CAD build for the part. Positions are in the model's coordinates, mm. A direction names the side the tool comes from. Round coordinates to 2 decimals unless told otherwise and drop trailing zeros. Loops run counter-clockwise (first coordinate to the right, second up) from the corner with the lowest first, then second, coordinate; pieces in that order, holes last. Notation, with made-up numbers: M 14.25,-4.5 L 25.25,-4.5 A23 ccw 25.25,13.5 Z; hole C 16.5,-30 d7. An arc over 180 degrees is marked long. Use a Markdown table: item, result. Add a question column.
(1) Band-saw the part on D-D, the plane z = 10.75. Give the number of separate pieces and of enclosed holes in the cut face, and give its area (3 significant figures).
(2) Flat gauge pins, fed straight in: P1, Ø3, axis at x = -8.5, y = -8.5, coming from the +Z side; P2, Ø2, axis at x = -14, z = 9.5, coming from the -Y side; P3, Ø5, axis at y = -9, z = 7, coming from the +X side. Where does each tip first touch, or does it go through?
(3) Band-saw the part on C-C, the plane y = 15. Write the cut outline in (x, z).
(4) Which spindle directions (+Z, -Z, +X, -X, +Y, -Y) get a long thin tool onto all of the face, cutting with end or side? Do faces 1 (the face through (9, -8.16, 1.87)), 2 (the face through (-23.65, -12.07, 4.76)), 3 (the face through (0.6, 9.7, 3.8)). Say none if no direction does.
(5) Wall check: L1, parallel to X at y = -0.5, z = 2; L2, parallel to X at y = 2, z = 5.5; L3, parallel to Y at x = 0.5, z = 1.25. Give the ranges that are in metal, low to high.
(6) Two-plate mould, pull along X, no slides. Class faces 4 (the face through (-28, 21, 7)), 5 (the face through (0, -7, 11.8)), 6 (the face through (-12.28, -0.06, 1.87)): released by +X, released by -X, zero draft, split by the parting line, or undercut.
(7) Band-saw the part on A-A, the plane y = 0. Write the cut outline in (x, z).
Autodesk Inventor part; units mm, degrees
ref_plane "YZ Plane" through (0, 0, 0) normal (1, 0, 0) x (0, 1, 0)
ref_plane "XZ Plane" through (0, 0, 0) normal (0, 1, 0) x (-1, 0, 0)
ref_plane "XY Plane" through (0, 0, 0) normal (0, 0, 1) x (1, 0, 0)
sketch "Эскиз1" plane through (0, 0, 0) normal (0, 0, 1) x (1, 0, 0)
  circle A0 centre (0, 0) radius 14
  circle A1 centre (-11, 0) radius 1.2813
  circle A2 centre (-7.7782, -7.7782) radius 1.2813
  circle A3 centre (0, -11) radius 1.2813
  circle A4 centre (7.7782, -7.7782) radius 1.2813
  circle A5 centre (11, 0) radius 1.2813
  circle A6 centre (7.7782, 7.7782) radius 1.2813
  circle A7 centre (0, 11) radius 1.2813
  circle A8 centre (-7.7782, 7.7782) radius 1.2813
  circle A9 centre (0, 0) radius 6
  dimension "d3" = 12
extrude "Выдавливание1" add sketch "Эскиз1" along normal blind 1.8
sketch "Эскиз2" plane through (0, 0, 1.8) normal (0, 0, 1) x (1, 0, 0)
  circle A0 centre (0, 0) radius 14
  circle A1 centre (0, 0) radius 6
  circle A2 centre (-7.7782, 7.7782) radius 1.2813
  circle A3 centre (0, 11) radius 1.2813
  circle A4 centre (7.7782, 7.7782) radius 1.2813
  circle A5 centre (11, 0) radius 1.2813
  circle A6 centre (7.7782, -7.7782) radius 1.2813
  circle A7 centre (0, -11) radius 1.2813
  circle A8 centre (-7.7782, -7.7782) radius 1.2813
  circle A9 centre (-11, 0) radius 1.2813
  circle A10 centre (0, 0) radius 35
  dimension "d4" = 70
extrude "Выдавливание2" add sketch "Эскиз2" along normal blind 10 contours A0 | A10
sketch "Эскиз3" plane through (0, 0, 11.8) normal (0, 0, 1) x (1, 0, 0)
  circle A0 centre (0, 11) radius 1.2813
  circle A1 centre (0, 11) radius 3
  point P0 (0, 0)
  dimension "d7" = 6
extrude "Выдавливание3" cut sketch "Эскиз3" against normal blind 8
pattern_circular "Круговой массив1" count 8 over 360 about axis through (0, 0, 0) along (0, 0, 1) of "Выдавливание3"
sketch "Эскиз4" plane through (0, 0, 1.8) normal (0, 0, -1) x (-1, 0, 0)
  circle A0 centre (-23, 15) radius 2
  point P0 (0, 0)
  dimension "d13" = 4
  dimension "d14" = 15
  dimension "d15" = 23
extrude "Выдавливание4" cut sketch "Эскиз4" against normal through all
sketch "Эскиз5" plane through (0, 0, 1.8) normal (0, 0, -1) x (-1, 0, 0)
  circle A0 centre (-23, 15) radius 2
  circle A1 centre (-23, 15) radius 3
  point P0 (0, 0)
  dimension "d18" = 6
extrude "Выдавливание5" cut sketch "Эскиз5" against normal blind 6 contours A0 | A1
mirror "Зеркальное отражение1" about plane through (0, 0, 0) normal (0, 1, 0) of "Выдавливание4", "Выдавливание5"
mirror "Зеркальное отражение2" about plane through (0, 0, 0) normal (1, 0, 0) of "Выдавливание4", "Выдавливание5", "Зеркальное отражение1"
properties part number "000.005.004.003 - ПОВОРОТНЫЙ ДИСК" material "Пластик АБС"
Return value:
| question | item | result |
|---|---|---|
| 1 | separate pieces | 1 |
| 1 | enclosed holes | 13 |
| 1 | area | 3,450 mm^2 |
| 2 | P1 | z = 3.8 |
| 2 | P2 | y = -32.5 |
| 2 | P3 | x = 34.39 |
| 3 | outline | M -31.62,1.8 L -26,1.8 L -26,7.8 L -25,7.8 L -25,11.8 L -31.62,11.8 Z; M -21,7.8 L -20,7.8 L -20,1.8 L 20,1.8 L 20,7.8 L 21,7.8 L 21,11.8 L -21,11.8 Z; M 25,7.8 L 26,7.8 L 26,1.8 L 31.62,1.8 L 31.62,11.8 L 25,11.8 Z |
| 4 | face 1 | +Z, -Z |
| 4 | face 2 | -Z |
| 4 | face 3 | +Z |
| 5 | L1 | -35 to -12.18, -9.82 to -5.98, 5.98 to 9.82, 12.18 to 35 |
| 5 | L2 | -34.94 to -13.24, -8.76 to -5.66, 5.66 to 8.76, 13.24 to 34.94 |
| 5 | L3 | -13.99 to -12.18, -9.82 to -5.98, 5.98 to 9.82, 12.18 to 13.99 |
| 6 | face 4 | split by the parting line |
| 6 | face 5 | zero draft |
| 6 | face 6 | undercut |
| 7 | outline | M -35,1.8 L -14,1.8 L -14,0 L -12.28,0 L -12.28,3.8 L -14,3.8 L -14,11.8 L -35,11.8 Z; M -9.72,0 L -6,0 L -6,11.8 L -8,11.8 L -8,3.8 L -9.72,3.8 Z; M 6,0 L 9.72,0 L 9.72,3.8 L 8,3.8 L 8,11.8 L 6,11.8 Z; M 12.28,0 L 14,0 L 14,1.8 L 35,1.8 L 35,11.8 L 14,11.8 L 14,3.8 L 12.28,3.8 Z |
